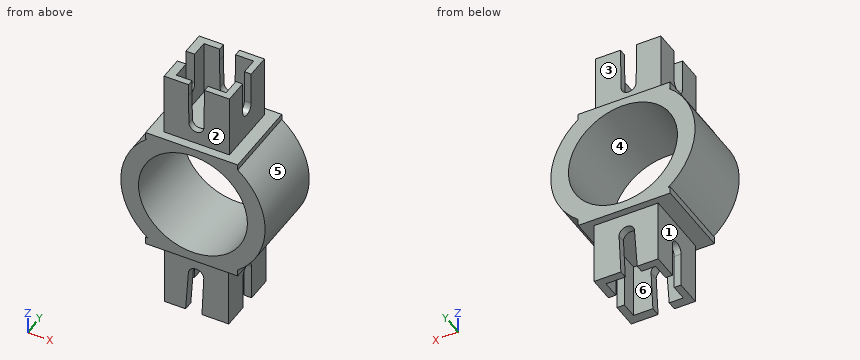
from build123d import *

# Parameters (mm, degrees)
F0_R      = 14.5
F0_R_2    = 10.95
F1_DEPTH  = 16
F2_W      = 18.492934294
F2_H      = 14.1721479595
F2_H_2    = 14.1267654391
F3_DEPTH  = 16
F4_W      = 10
F4_H      = 10
F5_DEPTH  = 11
F6_W      = 10
F6_H      = 10
F7_DEPTH  = 11
F9_DEPTH  = 25.4
F10_W     = 18.492934294
F10_H     = 16
F10_W_2   = 13.1218810566
F10_H_2   = 12.6919343169
F11_DEPTH = 12.7
F12_W     = 18.492934294
F12_H     = 16
F12_W_2   = 12.8853693604
F12_H_2   = 13.4778445354
F13_DEPTH = 12.7
F15_DEPTH = 25.4
F17_DEPTH = 25.4


with BuildPart() as f1:
    # F0 (on Front) → F1 (new body)
    with BuildSketch(Plane.XZ):
        Circle(F0_R)
        Circle(F0_R_2, mode=Mode.SUBTRACT)
    extrude(amount=F1_DEPTH)

    # F2 (on Front) → F3 (join)
    with BuildSketch(Plane.XZ):
        with Locations((-0.2633747645, 18.1480851024)):
            Rectangle(F2_W, F2_H)
        with Locations((-0.2633747645, -18.3736211107)):
            Rectangle(F2_W, F2_H_2)
    extrude(amount=F3_DEPTH)

    # F4 (on face) → F5 (cut)
    with BuildSketch(Plane.XY.offset(25.2341590822)):
        with Locations((0, -8)):
            Rectangle(F4_W, F4_H)
    extrude(amount=-F5_DEPTH, mode=Mode.SUBTRACT)

    # F6 (on face) → F7 (cut)
    with BuildSketch(Plane(origin=(0, 0, -25.4370038303), x_dir=(1, 0, 0), z_dir=(0, 0, -1))):
        with Locations((0.0633943081, 8)):
            Rectangle(F6_W, F6_H)
    extrude(amount=-F7_DEPTH, mode=Mode.SUBTRACT)

    # F8 (on face) → F9 (cut)
    with BuildSketch(Plane(origin=(0, 0, 0), x_dir=(-1, 0, 0), z_dir=(0, 1, 0))):
        with BuildLine():
            Line((1.8700940227, 22.6846607949), (1.8692923579, 22.6340436))
            ThreePointArc((1.8692923579, 22.6340436), (1.8698935939, 22.6593490235), (1.8700940227, 22.6846607949))
        make_face()
        with BuildLine():
            Line((1.7736972601, 16.5981590822), (1.8692923579, 22.6340436))
            Line((1.8692923579, 22.6340436), (1.8700940227, 22.6846607949))
            Line((1.8700940227, 22.6846607949), (1.8692926448, 22.7352689357))
            Line((1.8692926448, 22.7352689357), (1.8297228193, 25.2341590822))
            Line((1.8297228193, 25.2341590822), (-1.3672542312, 25.2341590822))
            Line((-1.3672542312, 25.2341590822), (-1.2305035169, 16.5981590822))
            ThreePointArc((-1.2305035169, 16.5981590822), (0.2715968716, 15.0960586937), (1.7736972601, 16.5981590822))
        make_face()
        with BuildLine():
            Line((1.8692926448, 22.7352689357), (1.8700940227, 22.6846607949))
            ThreePointArc((1.8700940227, 22.6846607949), (1.8698936656, 22.7099680376), (1.8692926448, 22.7352689357))
        make_face()
        with BuildLine():
            Line((2.097781384, -25.4370038303), (1.55, -17.0946339148))
            ThreePointArc((1.55, -17.0946339148), (0, -15.5446339148), (-1.55, -17.0946339148))
            Line((-1.55, -17.0946339148), (-1.5439814747, -17.2310934543))
            Line((-1.5439814747, -17.2310934543), (-1.1820611591, -25.4370038303))
            Line((-1.1820611591, -25.4370038303), (2.097781384, -25.4370038303))
        make_face()
        with BuildLine():
            Line((-1.5439814747, -17.2310934543), (-1.55, -17.0946339148))
            ThreePointArc((-1.55, -17.0946339148), (-1.5484946377, -17.1629300138), (-1.5439814747, -17.2310934543))
        make_face()
    extrude(amount=-F9_DEPTH, mode=Mode.SUBTRACT)

    # F10 (on face) → F11 (cut)
    with BuildSketch(Plane.XY.offset(25.2341590822)):
        with Locations((-0.2633747645, -8)):
            Rectangle(F10_W, F10_H)
        with Locations((-0.1905632671, -7.9240328416)):
            Rectangle(F10_W_2, F10_H_2, mode=Mode.SUBTRACT)
    extrude(amount=-F11_DEPTH, mode=Mode.SUBTRACT)

    # F12 (on face) → F13 (cut)
    with BuildSketch(Plane(origin=(0, 0, -25.4370038303), x_dir=(1, 0, 0), z_dir=(0, 0, -1))):
        with Locations((-0.2633747645, 8)):
            Rectangle(F12_W, F12_H)
        with Locations((0.125055667, 8.137495548)):
            Rectangle(F12_W_2, F12_H_2, mode=Mode.SUBTRACT)
    extrude(amount=-F13_DEPTH, mode=Mode.SUBTRACT)

    # F14 (on face) → F15 (cut)
    with BuildSketch(Plane.YZ.offset(6.3703772612)):
        with BuildLine():
            Line((-9.4740328416, 25.2341590822), (-9.4740328416, 18.6521150172))
            ThreePointArc((-9.4740328416, 18.6521150172), (-7.9240328416, 17.1021150172), (-6.3740328416, 18.6521150172))
            Line((-6.3740328416, 18.6521150172), (-6.3740328416, 25.2341590822))
            Line((-6.3740328416, 25.2341590822), (-9.4740328416, 25.2341590822))
        make_face()
    extrude(amount=-F15_DEPTH, mode=Mode.SUBTRACT)

    # F16 (on face) → F17 (cut)
    with BuildSketch(Plane(origin=(-6.3176290132, 0, 0), x_dir=(0, -1, 0), z_dir=(-1, 0, 0))):
        with BuildLine():
            Line((9.687495548, -25.4370038303), (9.687495548, -18.3815062046))
            ThreePointArc((9.687495548, -18.3815062046), (8.137495548, -16.8315062046), (6.587495548, -18.3815062046))
            Line((6.587495548, -18.3815062046), (6.587495548, -25.4370038303))
            Line((6.587495548, -25.4370038303), (9.687495548, -25.4370038303))
        make_face()
    extrude(amount=-F17_DEPTH, mode=Mode.SUBTRACT)


solid = f1.part
Here's how the part is built. I have some questions about the finished solid (model axes, mm). Face numbers are marked on the shaded views. A direction names the side the tool comes from. Coordinates: 2 decimals unless noted, no trailing zeros. Order: outer loops, then holes, each group sorted by start corner. A loop starts at its lowest first (then second) coordinate and runs counter-clockwise, first axis right, second up. Notation, with made-up numbers: M -32,68.25 L 26,68.25 A21 cw 26,93.25 Z; hole C -24.75,29 d9. An arc over 180 degrees is marked long. Answer as CSV lines item,"result". Start each with the question number.
1. I need wall thicknesses on line 1 (Z direction, x = 0, y = -8.5); line 2 (X direction, y = -4.25, z = -21.5); line 3 (Y direction, x = 6, z = -19). Which ranges of each line are inside material? Lowest first, please. Write a range as [from, to].
2. We'd pull the mould along Z, two halves only. Please class the marked faces 4, 5 and 6: released by +Z, released by -Z, zero draft, split by the parting line, or undercut.
3. I want a section at A-A, the plane z = 0. Write out the boundary of the cut face in (x, y), and give its area (3 significant figures).
4. For pin 1 (1 mm diameter, centred on y = -6.5, z = 8.5, fed in from +X); pin 2 (3 mm diameter, centred on x = 1.5, z = -20, fed in from +Y); pin 3 (6.5 mm diameter, centred on y = -6.5, z = 18.5, fed in from -X), each with a flat end and sliding along its axis, tell me the tip position at first contact or that it passes through.
5. On a 3-axis mill with a long thin cutter (end or side, diameter ignored), from which of +Z, -Z, +X, -X, +Y, -Y can I reach the whole of each face in a straight line? I mean the marked faces 1, 2 and 3. Say none if no direction works.
6. I want a section at B-B, the plane y = -10.5. Write out the boundary of the cut face in (x, z), and give its area (3 significant figures).
7. I want a section at D-D, the plane z = 7.5. Write out the boundary of the cut face in (x, y), and give its area (3 significant figures).
8. I want a section at C-C, the plane x = 3.5. Write out the boundary of the cut face in (y, z).
Recorded:
1,line 1,"z = [-14.44, -10.95], [10.95, 14.23]"
1,line 2,"x = [-6.32, -4.94], [5.06, 6.57]"
1,line 3,"y = [-14.88, -9.69], [-6.59, -1.4]"
2,face 4,"undercut"
2,face 5,"split by the parting line"
2,face 6,"zero draft"
3,outline,"M -14.5,-16 L -10.95,-16 L -10.95,0 L -14.5,0 Z; M 10.95,-16 L 14.5,-16 L 14.5,0 L 10.95,0 Z"
3,area,"114 mm2"
4,pin 1,"stops at x = 12.09"
4,pin 2,"stops at y = -1.4"
4,pin 3,"stops at x = -6.75"
5,face 1,"-Z, -X, +Y, -Y"
5,face 2,"+Z, +X, -X, -Y"
5,face 3,"+Z, +X, -X, +Y"
6,outline,"M -9.51,-12.74 L -6.32,-12.74 L -6.32,-25.44 L -4.94,-25.44 L -4.94,-14.44 L 5.06,-14.44 L 5.06,-25.44 L 6.57,-25.44 L 6.57,-12.74 L 8.98,-12.74 L 8.98,-11.38 A14.5 ccw 8.98,11.38 L 8.98,12.53 L 6.37,12.53 L 6.37,25.23 L 5,25.23 L 5,14.23 L -5,14.23 L -5,25.23 L -6.75,25.23 L -6.75,12.53 L -9.51,12.53 L -9.51,11.06 L -9.37,11.06 A14.5 ccw -9.07,-11.31 L -9.51,-11.31 Z; hole C 0,0 d21.9"
6,area,"364 mm2"
7,outline,"M -12.41,-16 L -7.98,-16 L -7.98,0 L -12.41,0 Z; M 7.98,-16 L 12.41,-16 L 12.41,0 L 7.98,0 Z"
7,area,"142 mm2"
8,outline,"M -16,-12.74 L -14.88,-12.74 L -14.88,-25.44 L -13,-25.44 L -13,-14.44 L -3,-14.44 L -3,-25.44 L -1.4,-25.44 L -1.4,-12.74 L 0,-12.74 L 0,-10.38 L -16,-10.38 Z; M -16,10.38 L 0,10.38 L 0,12.53 L -1.58,12.53 L -1.58,25.23 L -3,25.23 L -3,14.23 L -13,14.23 L -13,25.23 L -14.27,25.23 L -14.27,12.53 L -16,12.53 Z"
